Could you check a few things on this model? Use its own coordinates, in mm. A direction names the side the tool comes from. Round coordinates to 2 decimals unless told otherwise and drop trailing zeros. Loops run counter-clockwise (first coordinate to the right, second up) from the corner with the lowest first, then second, coordinate; pieces in that order, holes last. Notation, with made-up numbers: (39, 23) -> (76, 23) arc R17 cw to (76, 47) -> close; hole circle Ø11 at (84.5, -7.5). An arc over 180 degrees is marked (long way). One line per item, written item: value.
```python
from build123d import *

# Parameters (mm, degrees)
MODEL_R                 = 15
MODEL_R_2               = 1.5
SALIENTE_EXTRUIR1_DEPTH = 3


with BuildPart() as part:
    # Model → Saliente-Extruir1 (new body)
    with BuildSketch(Plane.XY):
        with Locations((215.747807914, 241.952019993)):
            Circle(MODEL_R)
        with Locations((215.747807914, 241.952019993)):
            Circle(MODEL_R_2, mode=Mode.SUBTRACT)
        with Locations((215.747807914, 232.952019993)):
            Circle(MODEL_R_2, mode=Mode.SUBTRACT)
        with Locations((215.747807914, 250.952019993)):
            Circle(MODEL_R_2, mode=Mode.SUBTRACT)
        with BuildLine():
            Line((223.122807913, 245.202019993), (221.372807913, 245.202019993))
            ThreePointArc((221.372807913, 245.202019993), (220.842477828, 244.982350079), (220.622807913, 244.452019993))
            Line((220.622807913, 244.452019993), (220.622807913, 239.452019993))
            ThreePointArc((220.622807913, 239.452019993), (220.842477828, 238.921689907), (221.372807913, 238.702019993))
            Line((221.372807913, 238.702019993), (223.122807913, 238.702019993))
            ThreePointArc((223.122807913, 238.702019993), (223.653137999, 238.921689907), (223.872807913, 239.452019993))
            Line((223.872807913, 239.452019993), (223.872807913, 244.452019993))
            ThreePointArc((223.872807913, 244.452019993), (223.653137999, 244.982350079), (223.122807913, 245.202019993))
        make_face(mode=Mode.SUBTRACT)
        with BuildLine():
            Line((208.372807913, 245.202019993), (210.122807913, 245.202019993))
            ThreePointArc((210.122807913, 245.202019993), (210.653137999, 244.982350079), (210.872807913, 244.452019993))
            Line((210.872807913, 244.452019993), (210.872807913, 239.452019993))
            ThreePointArc((210.872807913, 239.452019993), (210.653137999, 238.921689907), (210.122807913, 238.702019993))
            Line((210.122807913, 238.702019993), (208.372807913, 238.702019993))
            ThreePointArc((208.372807913, 238.702019993), (207.842477828, 238.921689907), (207.622807913, 239.452019993))
            Line((207.622807913, 239.452019993), (207.622807913, 244.452019993))
            ThreePointArc((207.622807913, 244.452019993), (207.842477828, 244.982350079), (208.372807913, 245.202019993))
        make_face(mode=Mode.SUBTRACT)
    extrude(amount=SALIENTE_EXTRUIR1_DEPTH)


solid = part.part
```
Item 1: For faces 1 (the face through (219, 242, 0)), 2 (the face through (209, 238.702, 1)), which set-ups out of +Z, -Z, +X, -X, +Y, -Y let a thin tool reach every point of the face, with its end or its side?
Output:
face 1: -Z, +X, -X, +Y, -Y
face 2: +Z, -Z
Item 2: If we section it at B-B on z = 1.55: List the corners of the cut face in (x, y) for me, plus the area to 3 significant figures.
Output:
outline: circle Ø30 at (215.75, 241.95); hole (207.62, 239.45) arc R0.75 ccw to (208.37, 238.7) -> (210.12, 238.7) arc R0.75 ccw to (210.87, 239.45) -> (210.87, 244.45) arc R0.75 ccw to (210.12, 245.2) -> (208.37, 245.2) arc R0.75 ccw to (207.62, 244.45) -> close; hole circle Ø3 at (215.75, 232.95); hole circle Ø3 at (215.75, 241.95); hole circle Ø3 at (215.75, 250.95); hole (220.62, 239.45) arc R0.75 ccw to (221.37, 238.7) -> (223.12, 238.7) arc R0.75 ccw to (223.87, 239.45) -> (223.87, 244.45) arc R0.75 ccw to (223.12, 245.2) -> (221.37, 245.2) arc R0.75 ccw to (220.62, 244.45) -> close
area: 644 mm²
Item 3: Will these pins go through, and if not, where does the flat tip stop? pin 1 Ø1.5 at (y, z) = (243, 2) entering from +X; pin 2 Ø1.5 at (x, z) = (220, 1.5) entering from -Y; pin 3 Ø4 at (x, y) = (215.75, 241.95) entering from -Z; pin 4 Ø2.5 at (x, y) = (215.75, 232.95) entering from +Z.
Output:
pin 1: stops at x = 230.74
pin 2: stops at y = 227.37
pin 3: stops at z = 0
pin 4: passes through
Item 4: If we section it at C-C on y = 244: List the corners of the cut face in (x, z) for me.
Output:
outline: (200.89, 0) -> (207.62, 0) -> (207.62, 3) -> (200.89, 3) -> close; (210.87, 0) -> (220.62, 0) -> (220.62, 3) -> (210.87, 3) -> close; (223.87, 0) -> (230.61, 0) -> (230.61, 3) -> (223.87, 3) -> close
Item 5: I need wall thicknesses on line 1 (X direction, y = 241.5, z = 0.7); line 2 (X direction, y = 244, z = 1.1); line 3 (Y direction, x = 222, z = 1.7). Which ranges of each line are inside material? Lowest first, please. Write a range as from..to.
Output:
line 1: x = 200.75..207.62, 210.87..214.32, 217.18..220.62, 223.87..230.74
line 2: x = 200.89..207.62, 210.87..220.62, 223.87..230.61
line 3: y = 228.32..238.7, 245.2..255.59
Item 6: If we mould it in two halves opening along Y, with no side actions, what happens to faces 3 (the face through (223.873, 242, 1)), 4 (the face through (213.795, 256.824, 1.479)), 5 (the face through (219, 242, 3))? For each: released by +Y, released by -Y, zero draft, split by the parting line, or undercut.
Output:
face 3: undercut
face 4: split by the parting line
face 5: zero draft
Item 7: If we section it at A-A on y = 233.5: List the corners of the cut face in (x, z) for me.
Output:
outline: (203.36, 0) -> (214.35, 0) -> (214.35, 3) -> (203.36, 3) -> close; (217.14, 0) -> (228.14, 0) -> (228.14, 3) -> (217.14, 3) -> close
Item 8: If we section it at D-D on x = 227.25: List the corners of the cut face in (y, z) for me.
Output:
outline: (232.32, 0) -> (251.58, 0) -> (251.58, 3) -> (232.32, 3) -> close
